```python
from build123d import *

# Parameters (mm, degrees)
CYLINDER001_R     = 3
CYLINDER001_DEPTH = 3
CYLINDER_R        = 1.9
CYLINDER_DEPTH    = 25


with BuildPart() as bolt_head:
    # Cylinder001 → Cylinder001 (new body)
    with BuildSketch(Plane.XY):
        Circle(CYLINDER001_R)
    extrude(amount=CYLINDER001_DEPTH)


with BuildPart() as m3_bolt:
    # Cylinder → Cylinder (new body)
    with BuildSketch(Plane.XY):
        Circle(CYLINDER_R)
    extrude(amount=CYLINDER_DEPTH)

    # Fusion: union Bolt_Head
    add(bolt_head.part)


solid = m3_bolt.part
```
Here's how the part is built. I have some questions about the finished solid (model axes, mm). A direction names the side the tool comes from. Give positions to 0.01 mm unless a question says otherwise; leave off trailing zeros. Loops run counter-clockwise (first coordinate to the right, second up) from the corner with the lowest first, then second, coordinate; pieces in that order, holes last. Notation, with made-up numbers: (14.5, 35.25) -> (52.5, 35.25) arc R21 ccw to (52.5, 67.25) -> close; hole circle Ø1 at (73, 77). An arc over 180 degrees is marked (long way). Use one line per item in the form item = value. Start each with the question number.
1) Imagine slicing it at C-C (z = 13.25). Please give me the cut outline in (x, y), then the cut area to 3 significant figures.
2) For P1, Ø1.5, axis at x = -1.5, y = -2, coming from the +Z side; P2, Ø1.5, axis at x = -1.5, z = 4.5, coming from the -Y side; P3, Ø1.5, axis at y = -1, z = 17.5, coming from the -X side, each with a flat end and sliding along its axis, tell me the tip position at first contact or that it passes through.
3) Imagine slicing it at D-D (y = 2.4). Please give me the cut outline in (x, z).
4) Please list where these lines run through material, in increasing order: line 1 along Z through (x, y) = (1.7, 2.05); line 2 along Y through (x, z) = (0.1, 16); line 3 along Y through (x, z) = (1.3, 18.25).
5) Imagine slicing it at A-A (y = 0). Please give me the cut outline in (x, z).
6) Which directions (+Z, -Z, +X, -X, +Y, -Y) give clear straight access to the entire face, cutting with the end or side of a thin tool? Please do faces 1 (the face through (-1.9, 0.08, 13.85)), 2 (the face through (0, 0, 0)).
Check values:
q1.outline = circle Ø3.8 at (0, 0)
q1.area = 11.3 mm^2
q2.P1 = 25
q2.P2 = -1.75
q2.P3 = -1.88
q3.outline = (-1.8, 0) -> (1.8, 0) -> (1.8, 3) -> (-1.8, 3) -> close
q4.line_1 = 0 to 3
q4.line_2 = -1.9 to 1.9
q4.line_3 = -1.39 to 1.39
q5.outline = (-3, 0) -> (3, 0) -> (3, 3) -> (1.9, 3) -> (1.9, 25) -> (-1.9, 25) -> (-1.9, 3) -> (-3, 3) -> close
q6.face_1 = +Z
q6.face_2 = -Z, +X, -X, +Y, -Y
